The drawing under review shows one solid part. Ordinate dimensions are in mm from its lowest x, y, z. Give positions to 0.01 mm unless a question says otherwise; leave off trailing zeros. Write each loop counter-clockwise with the first axis right and the second up, starting at its lowest first coordinate (ties: lowest second). Pieces come first, ordered by that corner, then holes. Notation, with made-up numbers: (-12.75, 68.5) -> (1.25, 68.5) arc R22 cw to (1.25, 75.5) -> close; hole circle Ø8 at (28, 4). An arc over 180 degrees is marked (long way). Use CSV: the item, a comma, the result in double quotes.
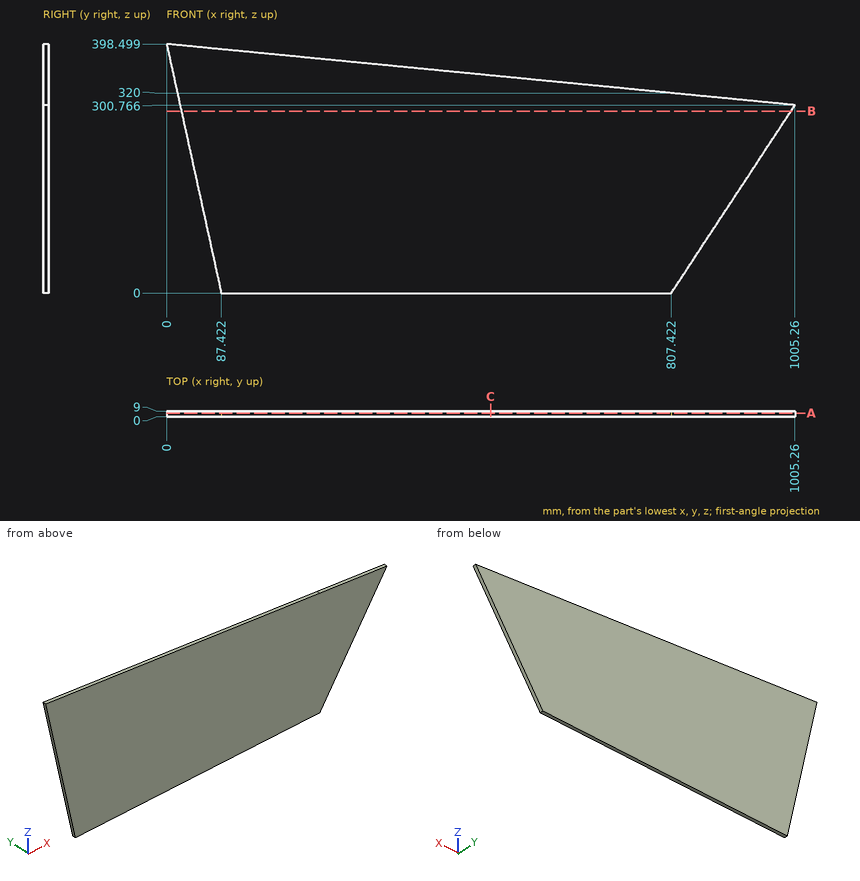
(1) Take a section at B-B (z = 291). Write out the cut boundary in (x, y).
Established:
outline,"(23.58, 0) -> (998.84, 0) -> (998.84, 9) -> (23.58, 9) -> close"
(2) Take a section at C-C (x = 518.5). Write out the cut boundary in (y, z), then the cut area to 3 significant figures.
Established:
outline,"(0, 0) -> (9, 0) -> (9, 348.09) -> (0, 348.09) -> close"
area,"3,130 mm2"
(3) Take a section at A-A (y = 5.75). Write out the cut boundary in (x, z) (1 decimal), then the cut area to 3 significant figures.
Established:
outline,"(0, 398.5) -> (87.4, 0) -> (807.4, 0) -> (1005.3, 300.8) -> close"
area,"304,000 mm2"
(4) Clearance check with flat-ended pins moving along their axes: pin 1 (3 mm diameter, centred on y = 5.5, z = 299.5, fed in from +X); pin 2 (3 mm diameter, centred on x = 680, y = 5, fed in from +Z); pin 3 (1 mm diameter, centred on y = 2, z = 265.5, fed in from +X); pin 4 (2 mm diameter, centred on y = 5, z = 153.5, fed in from -X). State where each tip first meets the part, or that it passes through.
Established:
pin 1,"stops at x = 1005.26"
pin 2,"stops at z = 332.53"
pin 3,"stops at x = 982.39"
pin 4,"stops at x = 53.53"
(5) For line 1 along Z through (x, y) = (709.5, 7); line 2 along Z through (x, y) = (216, 8.5); line 3 along X through (y, z) = (5.5, 125.5) (1 decimal), list the stretches that pass through material, from the lowest coordinate up. Write a range as [from, to].
Established:
line 1,"z = [0, 329.52]"
line 2,"z = [0, 377.5]"
line 3,"x = [59.9, 890]"
